```python
from build123d import *

# Parameters (mm, degrees)
SKETCH2_R               = 55.88
SKETCH2_R_2             = 44.45
BASE_CYLINDER_DEPTH     = 88.9
SKETCH3_R               = 63.5
SKETCH3_R_2             = 44.45
AFT_FLANGE_DEPTH        = 88.9
SKETCH6_R               = 50.9524
SKETCH6_R_2             = 47.4218
AFT_O_RING_DEPTH        = 1.9812
SKETCH_FOR_BOLT_HOLES_R = 3.2639
CUT_EXTRUDE1_DEPTH      = 89.9
SKETCH51_R              = 2.413
CUT_EXTRUDE2_DEPTH      = 4.826


with BuildPart() as part:
    # Sketch2 → Base Cylinder (new body)
    with BuildSketch(Plane(origin=(0, 0, 0), x_dir=(1, 0, 0), z_dir=(0, 1, 0))):
        Circle(SKETCH2_R)
        Circle(SKETCH2_R_2, mode=Mode.SUBTRACT)
    extrude(amount=BASE_CYLINDER_DEPTH)

    # Sketch3 → Aft Flange (add)
    with BuildSketch(Plane.XZ):
        Circle(SKETCH3_R)
        Circle(SKETCH3_R_2, mode=Mode.SUBTRACT)
    extrude(amount=-AFT_FLANGE_DEPTH)

    # Sketch6 → Aft O-Ring (cut)
    with BuildSketch(Plane.XZ):
        Circle(SKETCH6_R)
        Circle(SKETCH6_R_2, mode=Mode.SUBTRACT)
    extrude(amount=-AFT_O_RING_DEPTH, mode=Mode.SUBTRACT)

    # Sketch For Bolt Holes → Cut-Extrude1 (cut, through all)
    with BuildSketch(Plane.XZ):
        with Locations((15.120208615, 56.429386772)):
            Circle(SKETCH_FOR_BOLT_HOLES_R)
        with Locations((41.309178157, 41.309178157)):
            Circle(SKETCH_FOR_BOLT_HOLES_R)
        with Locations((56.429386772, 15.120208615)):
            Circle(SKETCH_FOR_BOLT_HOLES_R)
        with Locations((56.429386772, -15.120208615)):
            Circle(SKETCH_FOR_BOLT_HOLES_R)
        with Locations((41.309178157, -41.309178157)):
            Circle(SKETCH_FOR_BOLT_HOLES_R)
        with Locations((15.120208615, -56.429386772)):
            Circle(SKETCH_FOR_BOLT_HOLES_R)
        with Locations((-15.120208615, -56.429386772)):
            Circle(SKETCH_FOR_BOLT_HOLES_R)
        with Locations((-41.309178157, -41.309178157)):
            Circle(SKETCH_FOR_BOLT_HOLES_R)
        with Locations((-56.429386772, -15.120208615)):
            Circle(SKETCH_FOR_BOLT_HOLES_R)
        with Locations((-56.429386772, 15.120208615)):
            Circle(SKETCH_FOR_BOLT_HOLES_R)
        with Locations((-41.309178157, 41.309178157)):
            Circle(SKETCH_FOR_BOLT_HOLES_R)
        with Locations((-15.120208615, 56.429386772)):
            Circle(SKETCH_FOR_BOLT_HOLES_R)
    extrude(amount=-CUT_EXTRUDE1_DEPTH, mode=Mode.SUBTRACT)

    # Sketch51 → Cut-Extrude2 (cut)
    with BuildSketch(Plane(origin=(0, 88.9, 0), x_dir=(1, 0, 0), z_dir=(0, 1, 0))):
        with Locations((0, 58.42)):
            Circle(SKETCH51_R)
        with Locations((0, -58.42)):
            Circle(SKETCH51_R)
    extrude(amount=-CUT_EXTRUDE2_DEPTH, mode=Mode.SUBTRACT)


solid = part.part
```
Source: CAD feature listing. Evaluate the final solid. Frame: model axes, mm. A direction names the side the tool comes from. Round coordinates to 2 decimals unless told otherwise and drop trailing zeros. Loops run counter-clockwise (first coordinate to the right, second up) from the corner with the lowest first, then second, coordinate; pieces in that order, holes last.
1. Section query A-A on z = 0. Output: boundary loops of the cut face in (x, y).
2. Contact query for flat-ended pins moving along their axis: pin 1 (8.5 mm diameter, centred on x = 41.31, z = 41.31, fed in from +Y); pin 2 (10 mm diameter, centred on x = 21, y = 30.5, fed in from +Z); pin 3 (4 mm diameter, centred on x = 24.5, y = 23.5, fed in from -Z); pin 4 (6 mm diameter, centred on y = 52, z = -10, fed in from -X). Output: stop coordinate, or through.
3. Section query D-D on x = -42. Output: boundary loops of the cut face in (y, z).
4. Ray query, L1, parallel to Z at x = 0, y = 86.25; L2, parallel to X at y = 60, z = -55; L3, parallel to Z at x = -17.5, y = 70.5. Return the intervals inside material, ascending.
5. Section query C-C on y = 23.5. Give the number of separate pieces and of enclosed holes in the cut face, and give its area (3 significant figures).
6. Mould query, pull axis X, two halves, no side actions, for faces 4 (the cylindrical face through (14.413, 43.828, 53.243)), 5 (the cylindrical face through (-13.77, 43.83, -61.99)), 6 (the flat face through (0, 0, 52)). Classes: released by +X, released by -X, zero draft, split by the parting line, or undercut.
7. Section query B-B on x = 0. Output: boundary loops of the cut face in (y, z).
8. Access query for faces 1 (the cylindrical face through (-47.376, 0.977, 2.085)), 2 (the cylindrical face through (-0.523, 86.521, -56.064)), 3 (the cylindrical face through (-43.899, 43.828, 39.323)). Directions: +Z, -Z, +X, -X, +Y, -Y. A direction counts if a zero-diameter tool reaches every point of the face in a straight line with its end or side. Return the directions, or none.
Answers below:
1. outline: (-63.5, 0) - (-50.95, 0) - (-50.95, 1.98) - (-47.42, 1.98) - (-47.42, 0) - (-44.45, 0) - (-44.45, 88.9) - (-63.5, 88.9) - close; (44.45, 0) - (47.42, 0) - (47.42, 1.98) - (50.95, 1.98) - (50.95, 0) - (63.5, 0) - (63.5, 88.9) - (44.45, 88.9) - close
2. pin 1: stops at y = 88.9
2. pin 2: stops at z = 61.45
2. pin 3: stops at z = -59.38
2. pin 4: stops at x = -63.11
3. outline: (0, -47.63) - (88.9, -47.63) - (88.9, -44.5) - (0, -44.5) - close; (0, -38.12) - (88.9, -38.12) - (88.9, -14.55) - (0, -14.55) - (0, -22.02) - (1.98, -22.02) - (1.98, -28.85) - (0, -28.85) - close; (0, 14.55) - (88.9, 14.55) - (88.9, 38.12) - (0, 38.12) - (0, 28.85) - (1.98, 28.85) - (1.98, 22.02) - (0, 22.02) - close; (0, 44.5) - (88.9, 44.5) - (88.9, 47.63) - (0, 47.63) - close
4. L1: z = -63.5 to -60.83, -56.01 to -44.45, 44.45 to 56.01, 60.83 to 63.5
4. L2: x = -31.74 to -18.05, -12.19 to 12.19, 18.05 to 31.74
4. L3: z = -61.04 to -58.66, -54.2 to -40.86, 40.86 to 54.2, 58.66 to 61.04
5. separate pieces: 1
5. enclosed holes: 13
5. area: 6,060 mm2
6. face 4: undercut
6. face 5: split by the parting line
6. face 6: zero draft
7. outline: (0, -63.5) - (88.9, -63.5) - (88.9, -60.83) - (84.07, -60.83) - (84.07, -56.01) - (88.9, -56.01) - (88.9, -44.45) - (0, -44.45) - (0, -47.42) - (1.98, -47.42) - (1.98, -50.95) - (0, -50.95) - close; (0, 44.45) - (88.9, 44.45) - (88.9, 56.01) - (84.07, 56.01) - (84.07, 60.83) - (88.9, 60.83) - (88.9, 63.5) - (0, 63.5) - (0, 50.95) - (1.98, 50.95) - (1.98, 47.42) - (0, 47.42) - close
8. face 1: -Y
8. face 2: +Y
8. face 3: +Y, -Y
